Autodesk Inventor part; units mm, degrees
ref_plane "YZ Plane" through (0, 0, 0) normal (1, 0, 0) x (0, 1, 0)
ref_plane "XZ Plane" through (0, 0, 0) normal (0, 1, 0) x (-1, 0, 0)
ref_plane "XY Plane" through (0, 0, 0) normal (0, 0, 1) x (1, 0, 0)
sketch "Sketch1" plane through (0, 0, 0) normal (0, 1, 0) x (-1, 0, 0)
  line L0 (40, -40) -> (-40, -40) construction
  line L1 (-40, -40) -> (-40, 40) construction
  line L2 (-40, 40) -> (40, 40) construction
  line L3 (40, 40) -> (40, -40) construction
  line L4 (40, -40) -> (-40, 40) construction
  line L5 (-40, -40) -> (40, 40) construction
  circle A0 centre (-40, -40) radius 2.5
  arc A1 (-45.6569, -34.3431) -> (-34.3431, -45.6569) centre (-40, -40) ccw
  line L6 (-45.6569, -34.3431) -> (-35, -23.6863) construction
  line L7 (-35, -23.6863) -> (-35, 0) construction
  spline S0 degree 2 poles (-45.6569, -34.3431) (-35, -23.6863) (-35, 0) knots 1 1 1 2 2 2
  line L8 (-34.3431, -45.6569) -> (-45.6569, -34.3431) construction
  circle A2 centre (0, 0) radius 22.5
  line L9 (-34.3431, -45.6569) -> (-23.6863, -35) construction
  line L10 (-23.6863, -35) -> (0, -35) construction
  spline S1 degree 2 poles (-34.3431, -45.6569) (-23.6863, -35) (0, -35) knots 1 1 1 2 2 2
  line L11 (0, 0) -> (0, -47.3827) construction
  line L12 (0, 0) -> (-76.4691, 0) construction
  circle A3 centre (-40, 40) radius 2.5
  arc A4 (-34.3431, 45.6569) -> (-45.6569, 34.3431) centre (-40, 40) ccw
  line L13 (-45.6569, 34.3431) -> (-35, 23.6863) construction
  line L14 (-35, 23.6863) -> (-35, 0) construction
  spline S2 degree 2 poles (-45.6569, 34.3431) (-35, 23.6863) (-35, 0) knots 1 1 1 2 2 2
  spline S3 degree 2 poles (-34.3431, 45.6569) (-23.6863, 35) (0, 35) knots 1 1 1 2 2 2
  line L15 (-34.3431, 45.6569) -> (-23.6863, 35) construction
  line L16 (-23.6863, 35) -> (0, 35) construction
  circle A5 centre (40, -40) radius 2.5
  arc A6 (34.3431, -45.6569) -> (45.6569, -34.3431) centre (40, -40) ccw
  line L17 (45.6569, -34.3431) -> (35, -23.6863) construction
  line L18 (35, -23.6863) -> (35, 0) construction
  spline S4 degree 2 poles (45.6569, -34.3431) (35, -23.6863) (35, 0) knots 1 1 1 2 2 2
  spline S5 degree 2 poles (34.3431, -45.6569) (23.6863, -35) (0, -35) knots 1 1 1 2 2 2
  line L19 (34.3431, -45.6569) -> (23.6863, -35) construction
  line L20 (23.6863, -35) -> (0, -35) construction
  spline S6 degree 2 poles (45.6569, 34.3431) (35, 23.6863) (35, 0) knots 1 1 1 2 2 2
  arc A7 (45.6569, 34.3431) -> (34.3431, 45.6569) centre (40, 40) ccw
  circle A8 centre (40, 40) radius 2.5
  spline S7 degree 2 poles (34.3431, 45.6569) (23.6863, 35) (0, 35) knots 1 1 1 2 2 2
  line L21 (45.6569, 34.3431) -> (35, 23.6863) construction
  line L22 (35, 23.6863) -> (35, 0) construction
  line L23 (34.3431, 45.6569) -> (23.6863, 35) construction
  line L24 (23.6863, 35) -> (0, 35) construction
  dimension "d0" = 80
  dimension "d1" = 80
  dimension "d2" = 5
  dimension "d4" = 45
  dimension "d5" = 5
  dimension "d6" = 45
  dimension "d7" = 8
extrude "Extrusion1" add sketch "Sketch1" along normal blind 6
properties part number "YawBottomPlateThick"
Verification items for the finished model (mm, model axes). Give positions to 0.01 mm unless a question says otherwise; leave off trailing zeros. Answer as CSV lines item,"result". Start each with the question number.
Item 1: Section check A-A, the plane y = 2.5. State how many separate pieces and enclosed holes the cut face has, plus the area to 3 significant figures.
Item 2: Material ranges on L1, parallel to Z at x = -40, y = 1.95; L2, parallel to X at y = 4.5, z = -41.5; L3, parallel to Z at x = 10, y = 3, recorded low to high.
Item 3: Gauge pin test, flat ends, axial feed: pin 1 (1.5 mm diameter, centred on x = -24, y = 2, fed in from +Z); pin 2 (2 mm diameter, centred on x = 21, y = 2, fed in from +Z). Record the tip position at first contact, or that the pin passes through.
Item 4: Mould release check, pull along Z, two halves, no side actions. Record for faces 1 (the face through (37.69, 2.96, 40.96)), 2 (the face through (-21, 0, -10)): released by +Z, released by -Z, zero draft, split by the parting line, or undercut.
Filled in:
1,separate pieces,"1"
1,enclosed holes,"5"
1,area,"4,680 mm^2"
2,L1,"-48 to -42.5, -37.5 to -26.34, 26.34 to 37.5, 42.5 to 48"
2,L2,"-47.86 to -42, -38 to -29.05, 29.05 to 38, 42 to 47.86"
2,L3,"-35.54 to -20.16, 20.16 to 35.54"
3,pin 1,"z = 39.26"
3,pin 2,"z = 38.18"
4,face 1,"undercut"
4,face 2,"zero draft"
